Check sheet for the drawn part. Datum: minimum x, y, z corner. Units: mm. A direction names the side the tool comes from. Give positions to 0.01 mm unless a question says otherwise; leave off trailing zeros. Order: outer loops, then holes, each group sorted by start corner. A loop starts at its lowest first (then second) coordinate and runs counter-clockwise, first axis right, second up. Notation, with made-up numbers: (14.25, 63) -> (34.25, 63) arc R18 cw to (34.25, 81) -> close; hole circle Ø6 at (-14, 11.25). An arc over 180 degrees is marked (long way). One line per question, with ' | ' between items. Start each with the question number.
Q1. Material ranges on probe 1 along X at (y, z) = (39, 2) (1 decimal); probe 2 along Y at (x, z) = (22.75, 4.25); probe 3 along Y at (x, z) = (72, 5) (1 decimal), recorded low to high. Write a range as [from, to].
Q2. Section check D-D on z = 10.5. Record the cut outline in (x, y), plus the area to 3 significant figures.
Q3. Section check A-A on y = 39.25. Record the cut outline in (x, z), plus the area to 3 significant figures.
Q4. Access from +Z, -Z, +X, -X, +Y, -Y to the whole of each face (thin tool, end or side, straight path). Record for the marked faces 1, 2 and 3.
Q5. Section check C-C on z = 27. Record the cut outline in (x, y).
Q6. Go/stop test with flat-tipped pins: pin 1 (7 mm diameter, centred on y = 84, z = 8.5, fed in from -X); pin 2 (7 mm diameter, centred on x = 35.5, y = 81, fed in from +Z); pin 3 (1 mm diameter, centred on x = 8, z = 32.5, fed in from -Y); pin 4 (2 mm diameter, centred on x = 22.5, y = 10.5, fed in from -Z). Record where each tip stops, or that it passes through.
Q7. Section check B-B on z = 6. Give the number of separate pieces and of enclosed holes in the cut face, plus the area to 3 significant figures.
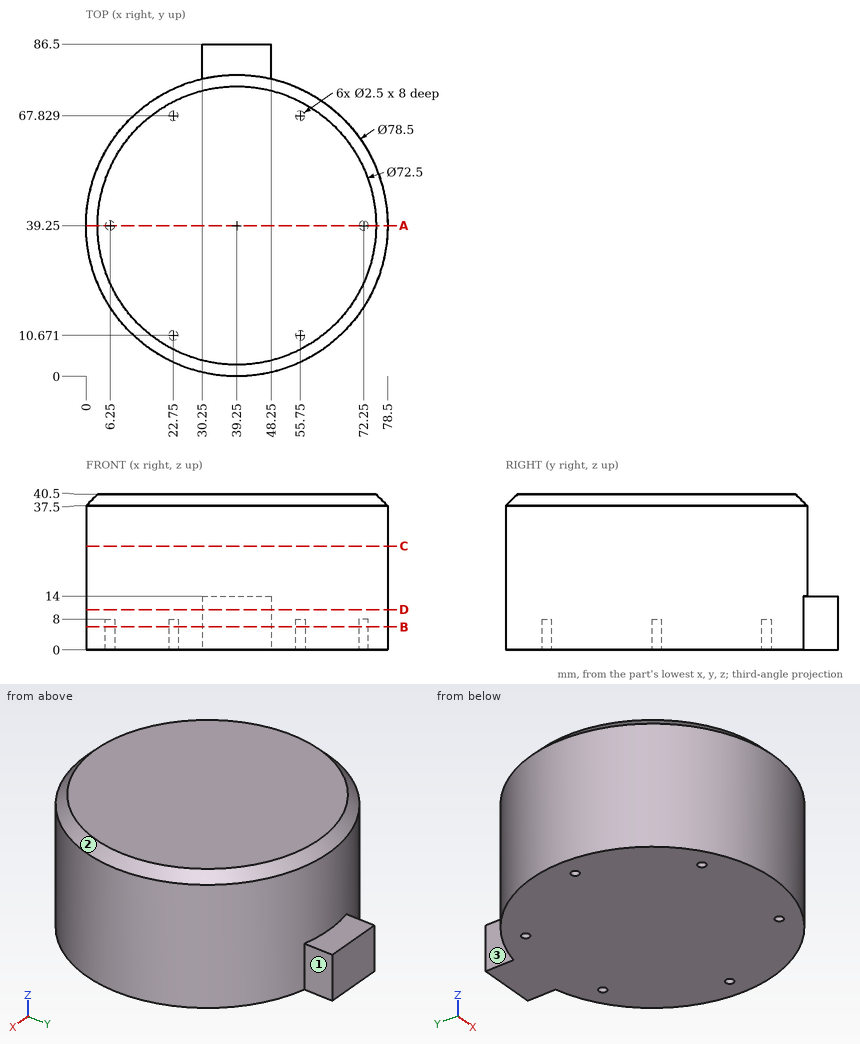
Filled in:
1) probe 1: [0, 5], [7.5, 71], [73.5, 78.5] | probe 2: [3.64, 9.42], [11.92, 66.58], [69.08, 74.86] | probe 3: [17.6, 38], [40.5, 60.9]
2) outline: (30.25, 77.45) arc R39.25 ccw (long way) to (48.25, 77.45) -> (48.25, 86.5) -> (30.25, 86.5) -> close | area: 4,990 mm²
3) outline: (0, 0) -> (5, 0) -> (5, 8) -> (7.5, 8) -> (7.5, 0) -> (71, 0) -> (71, 8) -> (73.5, 8) -> (73.5, 0) -> (78.5, 0) -> (78.5, 37.5) -> (75.5, 40.5) -> (3, 40.5) -> (0, 37.5) -> close | area: 3,130 mm²
4) face 1: +Z, -Z, +X, +Y | face 2: +Z | face 3: +Z, -Z, -X, +Y
5) outline: circle Ø78.5 at (39.25, 39.25)
6) pin 1: x = 30.25 | pin 2: z = 38.33 | pin 3: y = 14.86 | pin 4: z = 0
7) separate pieces: 1 | enclosed holes: 6 | area: 4,960 mm²
